```python
from build123d import *

# Parameters (mm, degrees)
F0_W     = 7.3
F0_H     = 3.5
F1_DEPTH = 19
F2_DEPTH = 1.5
F3_DEPTH = 10
F4_DEPTH = 4
F5_DEPTH = 1.5
F6_SIZE  = 0.5
F8_DEPTH = 6


with BuildPart() as f1:
    # F0 (on Top) → F1 (new body)
    with BuildSketch(Plane.XY):
        with BuildLine():
            ThreePointArc((7.3, -11.9461290802), (11.250406053, -8.3323684294), (13.5554417117, -3.5))
            Line((13.5554417117, -3.5), (7.3, -3.5))
            Line((7.3, -3.5), (7.3, -11.9461290802))
        make_face()
        with BuildLine():
            ThreePointArc((-7.3, -11.9461290802), (0, -14), (7.3, -11.9461290802))
            Line((7.3, -11.9461290802), (7.3, -3.5))
            Line((7.3, -3.5), (-7.3, -3.5))
            Line((-7.3, -3.5), (-7.3, -11.9461290802))
        make_face()
        with BuildLine():
            ThreePointArc((-13.5554417117, -3.5), (-11.250406053, -8.3323684294), (-7.3, -11.9461290802))
            Line((-7.3, -11.9461290802), (-7.3, -3.5))
            Line((-7.3, -3.5), (-13.5554417117, -3.5))
        make_face()
        with BuildLine():
            Line((-13.5554417117, -3.5), (-7.3, -3.5))
            Line((-7.3, -3.5), (-7.3, 0))
            Line((-7.3, 0), (-14, 0))
            ThreePointArc((-14, 0), (-13.8884157477, -1.7640600948), (-13.5554417117, -3.5))
        make_face()
        with BuildLine():
            Line((-14, 0), (-7.3, 0))
            Line((-7.3, 0), (-7.3, 3.5))
            Line((-7.3, 3.5), (-13.5554417117, 3.5))
            ThreePointArc((-13.5554417117, 3.5), (-13.8884157477, 1.7640600948), (-14, 0))
        make_face()
        with BuildLine():
            Line((-7.3, 3.5), (-7.3, 11.9461290802))
            ThreePointArc((-7.3, 11.9461290802), (-11.250406053, 8.3323684294), (-13.5554417117, 3.5))
            Line((-13.5554417117, 3.5), (-7.3, 3.5))
        make_face()
        with BuildLine():
            Line((7.3, 3.5), (7.3, 11.9461290802))
            ThreePointArc((7.3, 11.9461290802), (0, 14), (-7.3, 11.9461290802))
            Line((-7.3, 11.9461290802), (-7.3, 3.5))
            Line((-7.3, 3.5), (0, 3.5))
            Line((0, 3.5), (7.3, 3.5))
        make_face()
        with BuildLine():
            ThreePointArc((4.5, 8), (3.1819805153, 4.8180194847), (0, 3.5))
            ThreePointArc((0, 3.5), (-3.1819805153, 11.1819805153), (4.5, 8))
        make_face(mode=Mode.SUBTRACT)
        with BuildLine():
            Line((7.3, 3.5), (13.5554417117, 3.5))
            ThreePointArc((13.5554417117, 3.5), (11.250406053, 8.3323684294), (7.3, 11.9461290802))
            Line((7.3, 11.9461290802), (7.3, 3.5))
        make_face()
        with BuildLine():
            Line((7.3, 0), (14, 0))
            ThreePointArc((14, 0), (13.8884157477, 1.7640600948), (13.5554417117, 3.5))
            Line((13.5554417117, 3.5), (7.3, 3.5))
            Line((7.3, 3.5), (7.3, 0))
        make_face()
        with BuildLine():
            ThreePointArc((13.5554417117, -3.5), (13.8884157477, -1.7640600948), (14, 0))
            Line((14, 0), (7.3, 0))
            Line((7.3, 0), (7.3, -3.5))
            Line((7.3, -3.5), (13.5554417117, -3.5))
        make_face()
        Polygon((7.3, -3.5), (7.3, 0), (0, 0), (-7.3, 0), (-7.3, -3.5), align=None)
        with Locations((3.65, 1.75)):
            Rectangle(F0_W, F0_H)
        with Locations((-3.65, 1.75)):
            Rectangle(F0_W, F0_H)
        with BuildLine():
            ThreePointArc((4.5, 8), (-3.1819805153, 11.1819805153), (0, 3.5))
            ThreePointArc((0, 3.5), (3.1819805153, 4.8180194847), (4.5, 8))
        make_face()
        with BuildLine():
            ThreePointArc((2.5, 8), (1.767766953, 6.232233047), (0, 5.5))
            ThreePointArc((0, 5.5), (-1.767766953, 9.767766953), (2.5, 8))
        make_face(mode=Mode.SUBTRACT)
        with BuildLine():
            ThreePointArc((2.5, 8), (-1.767766953, 9.767766953), (0, 5.5))
            ThreePointArc((0, 5.5), (1.767766953, 6.232233047), (2.5, 8))
        make_face()
        with BuildLine():
            ThreePointArc((1.5, 8), (1.0606601718, 6.9393398282), (0, 6.5))
            ThreePointArc((0, 6.5), (-1.0606601718, 9.0606601718), (1.5, 8))
        make_face(mode=Mode.SUBTRACT)
        with BuildLine():
            ThreePointArc((1.5, 8), (-1.0606601718, 9.0606601718), (0, 6.5))
            ThreePointArc((0, 6.5), (1.0606601718, 6.9393398282), (1.5, 8))
        make_face()
        with BuildLine():
            Line((7.3, -17), (7.3, -11.9461290802))
            ThreePointArc((7.3, -11.9461290802), (0, -14), (-7.3, -11.9461290802))
            Line((-7.3, -11.9461290802), (-7.3, -17))
            Line((-7.3, -17), (7.3, -17))
        make_face()
    extrude(amount=-F1_DEPTH)

    # F0 (on Top) → F2 (join)
    with BuildSketch(Plane.XY):
        with BuildLine():
            Line((-17.5, 2.1), (-17.5, 3.5))
            ThreePointArc((-17.5, 3.5), (-21, 0), (-17.5, -3.5))
            Line((-17.5, -3.5), (-17.5, -2.1))
            ThreePointArc((-17.5, -2.1), (-19.6, 0), (-17.5, 2.1))
        make_face()
        with BuildLine():
            ThreePointArc((-17.5, -3.5), (-15.0251262658, -2.4748737342), (-14, 0))
            Line((-14, 0), (-15.4, 0))
            ThreePointArc((-15.4, 0), (-16.0150757595, -1.4849242405), (-17.5, -2.1))
            Line((-17.5, -2.1), (-17.5, -3.5))
        make_face()
        with BuildLine():
            Line((-17.5, -3.5), (-13.5554417117, -3.5))
            ThreePointArc((-13.5554417117, -3.5), (-13.8884157477, -1.7640600948), (-14, 0))
            ThreePointArc((-14, 0), (-15.0251262658, -2.4748737342), (-17.5, -3.5))
        make_face()
        with BuildLine():
            Line((-15.4, 0), (-14, 0))
            ThreePointArc((-14, 0), (-15.0251262658, 2.4748737342), (-17.5, 3.5))
            Line((-17.5, 3.5), (-17.5, 2.1))
            ThreePointArc((-17.5, 2.1), (-16.0150757595, 1.4849242405), (-15.4, 0))
        make_face()
        with BuildLine():
            ThreePointArc((-14, 0), (-13.8884157477, 1.7640600948), (-13.5554417117, 3.5))
            Line((-13.5554417117, 3.5), (-17.5, 3.5))
            ThreePointArc((-17.5, 3.5), (-15.0251262658, 2.4748737342), (-14, 0))
        make_face()
        with BuildLine():
            ThreePointArc((13.5554417117, 3.5), (13.8884157477, 1.7640600948), (14, 0))
            ThreePointArc((14, 0), (15.0251262658, 2.4748737342), (17.5, 3.5))
            Line((17.5, 3.5), (13.5554417117, 3.5))
        make_face()
        with BuildLine():
            ThreePointArc((17.5, -3.5), (15.0251262658, -2.4748737342), (14, 0))
            ThreePointArc((14, 0), (13.8884157477, -1.7640600948), (13.5554417117, -3.5))
            Line((13.5554417117, -3.5), (17.5, -3.5))
        make_face()
        with BuildLine():
            ThreePointArc((21, 0), (19.9748737342, 2.4748737342), (17.5, 3.5))
            Line((17.5, 3.5), (17.5, 2.1))
            ThreePointArc((17.5, 2.1), (18.9849242405, 1.4849242405), (19.6, 0))
            ThreePointArc((19.6, 0), (18.9849242405, -1.4849242405), (17.5, -2.1))
            Line((17.5, -2.1), (17.5, -3.5))
            ThreePointArc((17.5, -3.5), (19.9748737342, -2.4748737342), (21, 0))
        make_face()
        with BuildLine():
            Line((15.4, 0), (14, 0))
            ThreePointArc((14, 0), (15.0251262658, -2.4748737342), (17.5, -3.5))
            Line((17.5, -3.5), (17.5, -2.1))
            ThreePointArc((17.5, -2.1), (16.0150757595, -1.4849242405), (15.4, 0))
        make_face()
        with BuildLine():
            ThreePointArc((17.5, 3.5), (15.0251262658, 2.4748737342), (14, 0))
            Line((14, 0), (15.4, 0))
            ThreePointArc((15.4, 0), (16.0150757595, 1.4849242405), (17.5, 2.1))
            Line((17.5, 2.1), (17.5, 3.5))
        make_face()
    extrude(amount=-F2_DEPTH)

    # F0 (on Top) → F3 (join)
    with BuildSketch(Plane.XY):
        with BuildLine():
            ThreePointArc((1.5, 8), (-1.0606601718, 9.0606601718), (0, 6.5))
            ThreePointArc((0, 6.5), (1.0606601718, 6.9393398282), (1.5, 8))
        make_face()
    extrude(amount=F3_DEPTH)

    # F0 (on Top) → F4 (join)
    with BuildSketch(Plane.XY):
        with BuildLine():
            ThreePointArc((2.5, 8), (-1.767766953, 9.767766953), (0, 5.5))
            ThreePointArc((0, 5.5), (1.767766953, 6.232233047), (2.5, 8))
        make_face()
        with BuildLine():
            ThreePointArc((1.5, 8), (1.0606601718, 6.9393398282), (0, 6.5))
            ThreePointArc((0, 6.5), (-1.0606601718, 9.0606601718), (1.5, 8))
        make_face(mode=Mode.SUBTRACT)
    extrude(amount=F4_DEPTH)

    # F0 (on Top) → F5 (join)
    with BuildSketch(Plane.XY):
        with BuildLine():
            ThreePointArc((4.5, 8), (-3.1819805153, 11.1819805153), (0, 3.5))
            ThreePointArc((0, 3.5), (3.1819805153, 4.8180194847), (4.5, 8))
        make_face()
        with BuildLine():
            ThreePointArc((2.5, 8), (1.767766953, 6.232233047), (0, 5.5))
            ThreePointArc((0, 5.5), (-1.767766953, 9.767766953), (2.5, 8))
        make_face(mode=Mode.SUBTRACT)
    extrude(amount=F5_DEPTH)

    # F6
    f6_edges = [f1.edges().sort_by_distance(p)[0] for p in [
        (0, 9.5, 10),
    ]]
    chamfer(f6_edges, length=F6_SIZE)

    # F7 (on face) → F8 (cut)
    with BuildSketch(Plane.XY.offset(10)):
        Polygon((0, 9), (1.5, 9), (1.5, 9.5), (-1.5, 9.5), (-1.5, 9), align=None)
        Polygon((1.5, 6.5), (1.5, 7), (0, 7), (-1.5, 7), (-1.5, 6.5), align=None)
    extrude(amount=-F8_DEPTH, mode=Mode.SUBTRACT)


solid = f1.part
```
Check sheet for the modelled part. Datum: model origin and axes. Units: mm. A direction names the side the tool comes from. Coordinates: 2 decimals unless noted, no trailing zeros. Write each loop counter-clockwise with the first axis right and the second up, starting at its lowest first coordinate (ties: lowest second). Pieces come first, ordered by that corner, then holes. Notation, with made-up numbers: (21, 12) - (69, 12) arc R4 ccw to (69, 19) - close; hole circle Ø4 at (51.25, 75.5). An arc over 180 degrees is marked (long way). One line per question, with ' | ' between items.
Item 1: Sectioned sample at C-C on x = -4. Record the boundary of the cut face in (y, z), plus the area to 3 significant figures.
Determined:
outline: (-17, -19) - (13.42, -19) - (13.42, 0) - (10.06, 0) - (10.06, 1.5) - (5.94, 1.5) - (5.94, 0) - (-17, 0) - close | area: 584 mm2
Item 2: Access from +Z, -Z, +X, -X, +Y, -Y to the whole of each face (thin tool, end or side, straight path). Record for faces 1 (the face through (0, 7, 7)), 2 (the face through (-16, 3.5, -1)), 3 (the face through (16, -3.5, -1)).
Determined:
face 1: +Z, +X, -X, -Y | face 2: +Z, -Z, -X, +Y | face 3: +Z, -Z, +X, -Y
Item 3: Sectioned sample at B-B on z = 8. Record the boundary of the cut face in (x, y).
Determined:
outline: (-1.12, 7) - (1.12, 7) arc R1.5 ccw to (1.12, 9) - (-1.12, 9) arc R1.5 ccw to start
Item 4: Sectioned sample at D-D on z = -10. Record the boundary of the cut face in (x, y), plus the area to 3 significant figures.
Determined:
outline: (-7.3, -17) - (7.3, -17) - (7.3, -11.95) arc R14 ccw (long way) to (-7.3, -11.95) - close | area: 669 mm2
Item 5: Gauge pin test, flat ends, axial feed: P1, Ø1.5, axis at y = -13.5, z = -14, coming from the -X side; P2, Ø6, axis at x = -3.5, z = -11.5, coming from the +Y side; P3, Ø12, axis at x = -5.5, y = 1, coming from the +Z side; P4, Ø12, axis at x = -16.5, y = -5.5, coming from the -Z side. Record the tip position at first contact, or that the pin passes through.
Determined:
P1: stops at x = -7.3 | P2: stops at y = 13.99 | P3: stops at z = 1.5 | P4: stops at z = -19
Item 6: Sectioned sample at A-A on x = 18. Record the boundary of the cut face in (y, z).
Determined:
outline: (-3.46, -1.5) - (-2.04, -1.5) - (-2.04, 0) - (-3.46, 0) - close; (2.04, -1.5) - (3.46, -1.5) - (3.46, 0) - (2.04, 0) - close
Item 7: Thickness scan on line 1 (Z direction, x = -3, y = 0.5); line 2 (Z direction, x = 1, y = 9.5); line 3 (X direction, y = -0.5, z = -4.25). Record the ranges inside material, lowest first. Write a range as [from, to].
Determined:
line 1: z = [-19, 0] | line 2: z = [-19, 4] | line 3: x = [-13.99, 13.99]
